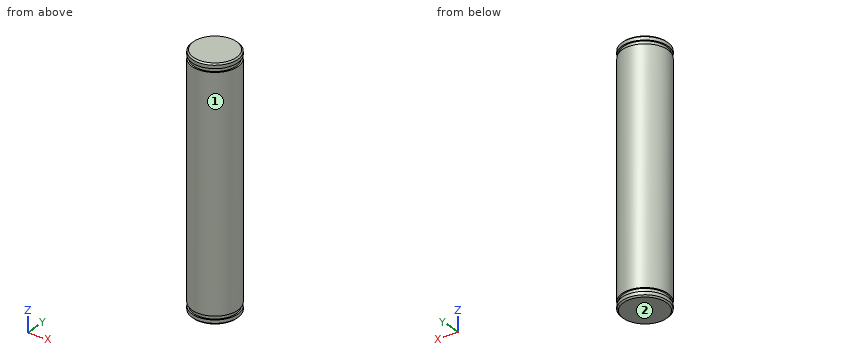
Autodesk Inventor part; units mm, degrees
ref_plane "YZ Plane" through (0, 0, 0) normal (1, 0, 0) x (0, 1, 0)
ref_plane "XZ Plane" through (0, 0, 0) normal (0, 1, 0) x (-1, 0, 0)
ref_plane "XY Plane" through (0, 0, 0) normal (0, 0, 1) x (1, 0, 0)
sketch "Sketch1" plane through (0, 0, 0) normal (0, 0, 1) x (1, 0, 0)
  circle A0 centre (0, 0) radius 6.35
  dimension "d0" = 12.7
extrude "Extrusion1" add sketch "Sketch1" along normal blind 31.75
sketch "Sketch6" plane through (0, 0, 31.75) normal (0, 0, 1) x (1, 0, 0)
  circle A0 centre (0, 0) radius 6.35
  circle A1 centre (0, 0) radius 5.9436
  dimension "d18" = 11.8872
extrude "Extrusion6" add sketch "Sketch6" along normal blind 0.9906 contours A1
sketch "Sketch7" plane through (0, 0, 32.7406) normal (0, 0, 1) x (1, 0, 0)
  circle A0 centre (0, 0) radius 6.35
extrude "Extrusion7" add sketch "Sketch7" along normal blind 1.27
chamfer "Chamfer1" distance 0.381 angle 45 1 edges at (-6.35, 0, 34.0106)
mirror "Mirror2" about plane through (0, 0, 0) normal (0, 0, -1)
properties part number "Carriage Shaft - Lower" material "Aluminum 6061"
For this review, take the finished solid that the model builds, in its own axes (mm). Face numbers are marked on the shaded views. Coordinates: 2 decimals unless noted, no trailing zeros. Loops run counter-clockwise (first coordinate to the right, second up) from the corner with the lowest first, then second, coordinate; pieces in that order, holes last. Notation, with made-up numbers: (19, 66) -> (60, 66) arc R18 ccw to (60, 80) -> close; hole circle Ø7 at (3, 64.5). An arc over 180 degrees is marked (long way). Write each question's results on one line, items separated by ' | '.
Q1. To check wall thickness, follow line 1 along Z through (x, y) = (-6, 1.75); line 2 along X through (y, z) = (-0.25, 18); line 3 along Y through (x, z) = (-1.75, -16.5). State the ranges of each line that lie inside material, in increasing order. Write a range as [from, to].
Taken from the geometry:
line 1: [-33.73, -32.74], [-31.75, 31.75], [32.74, 33.73] | line 2: [-6.35, 6.35] | line 3: [-6.1, 6.1]
Q2. Mouldability with a two-part tool opening along Y and no side actions: class the marked faces 1 and 2 as +Y half, -Y half, draft (parallel to the pull), parting line (faces both ways), or undercut.
Taken from the geometry:
face 1: parting line | face 2: draft
Q3. Add section A-A, the plane z = -22. State the section outline as (x, y) points, then the cut area to 3 significant figures.
Taken from the geometry:
outline: circle Ø12.7 at (0, 0) | area: 127 mm²
Q4. For pin 1 Ø3 at (y, z) = (-4, 24) entering from -X; pin 2 Ø1.5 at (y, z) = (2.5, 10.5) entering from -X; pin 3 Ø5 at (y, z) = (-4.5, -15) entering from -X, all flat-tipped, find the tip position at first contact; note any pin that passes through.
Taken from the geometry:
pin 1: x = -5.84 | pin 2: x = -6.1 | pin 3: x = -6.03
